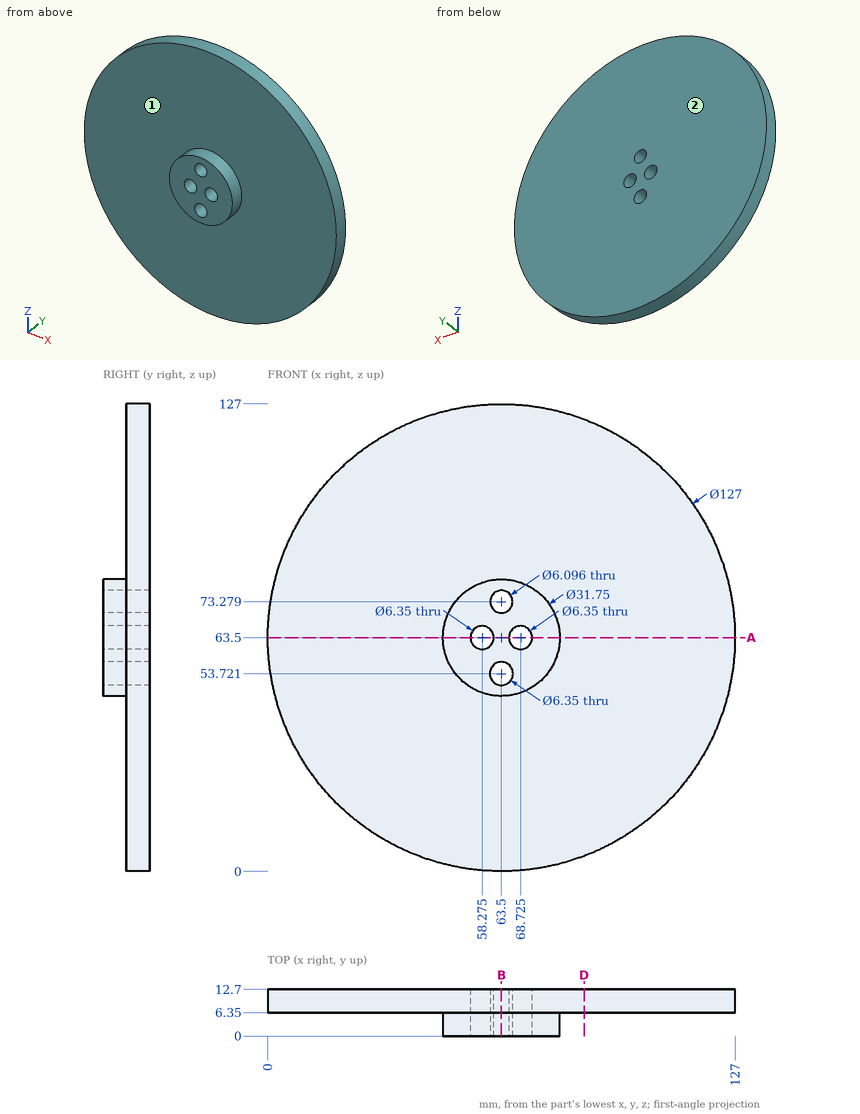
Part print with two shaded views. Sizes in mm from the minimum x, y, z corner. A direction names the side the tool comes from. Round coordinates to 2 decimals unless told otherwise and drop trailing zeros. Order: outer loops, then holes, each group sorted by start corner. A loop starts at its lowest first (then second) coordinate and runs counter-clockwise, first axis right, second up.
(1) Band-saw the part on D-D (x = 86). List the corners of the cut face in (y, z), then the cut area to 3 significant figures.
(2) 3-axis set-ups, long thin cutter, end or side, ignore diameter. For the marked faces 1 and 2: which of +Z, -Z, +X, -X, +Y, -Y reach the whole face in a straight line?
(3) Band-saw the part on A-A (z = 63.5). Give the number of separate pieces and of enclosed holes in the cut face, then the cut area to 3 significant figures.
(4) Band-saw the part on B-B (x = 63.5). List the corners of the cut face in (y, z) (3 decimals).
(5) Drill centre lines: line 1 (Z direction, x = 63.5, y = 6.25) (3 decimals); line 2 (Z direction, x = 64.5, y = 1.25) (1 decimal); line 3 (Y direction, x = 74.5, z = 107.5). Where is each one in solid material? Low to high.
(6) Pin check, flat tips, straight feed: pin 1 (3 mm diameter, centred on x = 100.5, z = 87.5, fed in from -Y); pin 2 (6 mm diameter, centred on y = 7.5, z = 98.5, fed in from +X); pin 3 (3 mm diameter, centred on x = 40.5, y = 7, fed in from +Z); pin 4 (4 mm diameter, centred on x = 58.28, z = 63.5, fed in from -Y). Stop position of each tip, or through.
Verdict:
1. outline: (6.35, 4.12) - (12.7, 4.12) - (12.7, 122.88) - (6.35, 122.88) - close
1. area: 754 mm2
2. face 1: -Y
2. face 2: +Z, -Z, +X, -X, +Y
3. separate pieces: 3
3. enclosed holes: 0
3. area: 847 mm2
4. outline: (0, 47.625) - (6.35, 47.625) - (6.35, 0) - (12.7, 0) - (12.7, 50.546) - (0, 50.546) - close; (0, 56.896) - (12.7, 56.896) - (12.7, 70.231) - (0, 70.231) - close; (0, 76.327) - (12.7, 76.327) - (12.7, 127) - (6.35, 127) - (6.35, 79.375) - (0, 79.375) - close
5. line 1: z = 47.625 to 50.546, 56.896 to 70.231, 76.327 to 79.375
5. line 2: z = 47.7 to 50.7, 56.7 to 70.4, 76.2 to 79.3
5. line 3: y = 6.35 to 12.7
6. pin 1: stops at y = 6.35
6. pin 2: stops at x = 118.35
6. pin 3: stops at z = 123.25
6. pin 4: passes through
